For this review, take the finished solid that the model builds, in its own axes (mm). A direction names the side the tool comes from. Coordinates: 2 decimals unless noted, no trailing zeros. Order: outer loops, then holes, each group sorted by start corner. A loop starts at its lowest first (then second) coordinate and runs counter-clockwise, first axis right, second up. Notation, with made-up numbers: (30, -15.5) - (37, -15.5) arc R14 cw to (37, -3.5) - close; hole circle Ø11 at (17.25, -9.5). An arc over 180 degrees is marked (long way). One line per item, written item: value. Start each with the question number.
(1) Consider section C-C on x = -58. Write out the cut boundary in (y, z), then the cut area to 3 significant figures.
(2) Consider section B-B on z = 39. Write out the cut boundary in (x, y).
(3) Consider section A-A on y = 85. Write out the cut boundary in (x, z), then the cut area to 3 significant figures.
(4) Mouldability with a two-part tool opening along X and no side actions: class faces 6 (the cylindrical face through (-31.8, 141.5, -37.1)), 7 (the flat face through (-11, 186.597, 22)), 8 (the cylindrical face through (-8.52, 6.23, 2.79)), 9 (the flat face through (0, 92, 1)) as released by +X, released by -X, zero draft, split by the parting line, or undercut.
(5) To check wall thickness, follow line 1 along X through (y, z) = (146, 39); line 2 along X through (y, z) = (71, -7); line 3 along Y through (x, z) = (-84, 0). State the ranges of each line that lie inside material, in increasing order.
(6) Clearance check with flat-ended pins moving along their axes: pin 1 (2.5 mm diameter, centred on y = 11.6, z = 12, fed in from +X); pin 2 (10.5 mm diameter, centred on y = 169.5, z = 33.5, fed in from +X); pin 3 (5 mm diameter, centred on x = -39.5, z = 11.5, fed in from -Y); pin 4 (3 mm diameter, centred on x = -46.5, z = 38.5, fed in from +Y). State where each tip first meets the part, or that it passes through.
(7) For faces 1 (the flat face through (-8, 169, 23)), 2 (the flat face through (-48, 99, 15)), 3 (the flat face through (-10, 47, 0)), 4 (the flat face through (-45, 98, -15)), 5 (the flat face through (-11, 169, 45)), list the 3-axis set-ups (+Z, -Z, +X, -X, +Y, -Y) from which the entire face can be reached by the end or side of a thin tool; tool diameter is ignored.
(8) Consider section D-D on z = -39. Write out the cut boundary in (x, y), then the cut area to 3 significant figures.
```python
from build123d import *

# Parameters (mm, degrees)
BOSS_EXTRUDE1_DEPTH = 10
SKETCH4_W           = 30
SKETCH4_H           = 15
BOSS_EXTRUDE2_DEPTH = 70
BOSS_EXTRUDE3_DEPTH = 10
SKETCH6_R           = 6.05
CUT_EXTRUDE3_DEPTH  = 3
SKETCH7_R           = 1.025
CUT_EXTRUDE4_DEPTH  = 139.126108227
SKETCH10_R          = 1.5
CUT_EXTRUDE9_DEPTH  = 10
BOSS_EXTRUDE4_DEPTH = 90
SKETCH15_W          = 5.5
SKETCH15_H          = 45
BOSS_EXTRUDE5_DEPTH = 35
SKETCH16_R          = 6.5
CUT_EXTRUDE10_DEPTH = 5.5
SKETCH17_R          = 2
CUT_EXTRUDE11_DEPTH = 34


with BuildPart() as part:
    # Sketch1 → Boss-Extrude1 (new body)
    with BuildSketch(Plane(origin=(0, 0, 0), x_dir=(0, 0, -1), z_dir=(1, 0, 0))):
        with BuildLine():
            Line((15, 11.596692486), (15, 111.596692486))
            Line((15, 111.596692486), (-15, 111.596692486))
            Line((-15, 111.596692486), (-15, 11.596692486))
            ThreePointArc((-15, 11.596692486), (0, -3.403307514), (15, 11.596692486))
        make_face()
    extrude(amount=-BOSS_EXTRUDE1_DEPTH)

    # Sketch4 → Boss-Extrude2 (add)
    with BuildSketch(Plane.ZY.offset(10)):
        with Locations((0, 104.096692486)):
            Rectangle(SKETCH4_W, SKETCH4_H)
    extrude(amount=BOSS_EXTRUDE2_DEPTH)

    # Sketch5 → Boss-Extrude3 (add)
    with BuildSketch(Plane.ZY.offset(80)):
        with BuildLine():
            Line((-15, 111.596692486), (15, 111.596692486))
            Line((15, 111.596692486), (15, 11.596692486))
            ThreePointArc((15, 11.596692486), (0, -3.403307514), (-15, 11.596692486))
            Line((-15, 11.596692486), (-15, 111.596692486))
        make_face()
    extrude(amount=BOSS_EXTRUDE3_DEPTH)

    # Sketch6 → Cut-Extrude3 (cut)
    with BuildSketch(Plane.ZY.offset(10)):
        with Locations((0, 11.596692486)):
            Circle(SKETCH6_R)
    extrude(amount=-CUT_EXTRUDE3_DEPTH, mode=Mode.SUBTRACT)

    # Sketch7 → Cut-Extrude4 (cut, through all)
    with BuildSketch(Plane.ZY.offset(10)):
        with Locations((0, 23.596692486)):
            Circle(SKETCH7_R)
        with Locations((12, 11.596692486)):
            Circle(SKETCH7_R)
        with Locations((0, -0.403307514)):
            Circle(SKETCH7_R)
        with Locations((-12, 11.596692486)):
            Circle(SKETCH7_R)
        with Locations((0, 11.596692486)):
            Circle(SKETCH7_R)
    extrude(amount=-CUT_EXTRUDE4_DEPTH, mode=Mode.SUBTRACT)

    # Sketch10 → Cut-Extrude9 (cut)
    with BuildSketch(Plane.ZY.offset(90)):
        with Locations((0, 11.596692486)):
            Circle(SKETCH10_R)
    extrude(amount=-CUT_EXTRUDE9_DEPTH, mode=Mode.SUBTRACT)

    # Sketch14 → Boss-Extrude4 (add)
    with BuildSketch(Plane.ZY.offset(90)):
        Polygon((-15, 111.596692486), (-60, 151.596692486), (60, 151.596692486), (15, 111.596692486), align=None)
    extrude(amount=-BOSS_EXTRUDE4_DEPTH)

    # Sketch15 → Boss-Extrude5 (add)
    with BuildSketch(Plane(origin=(0, 151.596692486, 0), x_dir=(1, 0, 0), z_dir=(0, 1, 0))):
        with Locations((-10.75, -22.5)):
            Rectangle(SKETCH15_W, SKETCH15_H)
    extrude(amount=BOSS_EXTRUDE5_DEPTH)

    # Sketch16 → Cut-Extrude10 (cut)
    with BuildSketch(Plane(origin=(-8, 0, 0), x_dir=(0, 0, -1), z_dir=(1, 0, 0))):
        with Locations((-14.7, 171.596692486)):
            Circle(SKETCH16_R)
    extrude(amount=-CUT_EXTRUDE10_DEPTH, mode=Mode.SUBTRACT)

    # Sketch17 → Cut-Extrude11 (cut)
    with BuildSketch(Plane(origin=(0, 151.596692486, 0), x_dir=(1, 0, 0), z_dir=(0, 1, 0))):
        with Locations(Location((-32.421605661, 39, 0), (0, 0, 270))):
            Circle(SKETCH17_R)
        with Locations(Location((-32.421605661, -39, 0), (0, 0, 270))):
            Circle(SKETCH17_R)
    extrude(amount=-CUT_EXTRUDE11_DEPTH, mode=Mode.SUBTRACT)


solid = part.part
```
Geometry check:
1. outline: (96.6, -15) - (111.6, -15) - (151.6, -60) - (151.6, 60) - (111.6, 15) - (96.6, 15) - close
1. area: 3,450 mm^2
2. outline: (-90, 132.93) - (-34.42, 132.93) - (-34.42, 151.6) - (-90, 151.6) - close; (-30.42, 132.93) - (0, 132.93) - (0, 151.6) - (-8, 151.6) - (-8, 186.6) - (-13.5, 186.6) - (-13.5, 151.6) - (-30.42, 151.6) - close
3. outline: (-90, -15) - (-80, -15) - (-80, 15) - (-90, 15) - close; (-10, -15) - (0, -15) - (0, 15) - (-10, 15) - close
3. area: 600 mm^2
4. face 6: undercut
4. face 7: zero draft
4. face 8: undercut
4. face 9: released by +X
5. line 1: x = -90 to -34.42, -30.42 to 0
5. line 2: x = -90 to -80, -10 to 0
5. line 3: y = -3.4 to 10.1, 13.1 to 151.6
6. pin 1: stops at x = 0
6. pin 2: stops at x = -8
6. pin 3: stops at y = 96.6
6. pin 4: stops at y = 151.6
7. face 1: +Z, -Z, +X, +Y
7. face 2: +Z, +X, -X, -Y
7. face 3: +Z, -Z, -Y
7. face 4: -Z, +X, -X, -Y
7. face 5: +Z, +X, -X, +Y
8. outline: (-90, 132.93) - (-34.42, 132.93) - (-34.42, 151.6) - (-90, 151.6) - close; (-30.42, 132.93) - (0, 132.93) - (0, 151.6) - (-30.42, 151.6) - close
8. area: 1,610 mm^2
